```python
from build123d import *

# Parameters (mm, degrees)
SKETCH1_R                = 155.575
SKETCH1_R_2              = 7.9375
BOSS_EXTRUDE1_DEPTH      = 4.7625
FILLET1_R                = 12.7
FILLET4_R                = 2.54
H_0_266_DIAMETER_HOLE1_D = 6.7564


with BuildPart() as part:
    # Sketch1 → Boss-Extrude1 (new body)
    with BuildSketch(Plane.XY):
        Circle(SKETCH1_R)
        with BuildLine():
            ThreePointArc((-125.107792883, -62.16212802), (-120.983748909, 69.85), (-8.719914422, 139.427590858))
            Line((-8.719914422, 139.427590858), (-12.49892387, 7.216257061))
            Line((-12.49892387, 7.216257061), (-125.107792883, -62.16212802))
        make_face(mode=Mode.SUBTRACT)
        with BuildLine():
            ThreePointArc((8.719914422, 139.427590858), (120.983748909, 69.85), (125.107792883, -62.16212802))
            Line((125.107792883, -62.16212802), (12.49892387, 7.216257061))
            Line((12.49892387, 7.216257061), (8.719914422, 139.427590858))
        make_face(mode=Mode.SUBTRACT)
        with BuildLine():
            ThreePointArc((116.38787846, -77.265462838), (0, -139.7), (-116.38787846, -77.265462838))
            Line((-116.38787846, -77.265462838), (0, -14.432514122))
            Line((0, -14.432514122), (116.38787846, -77.265462838))
        make_face(mode=Mode.SUBTRACT)
        with BuildLine():
            Line((-12.585726429, 4.179407795), (-12.694815268, 0.362857143))
            ThreePointArc((-12.694815268, 0.362857143), (-10.998522628, -6.35), (-6.03316413, -11.17546109))
            Line((-6.03316413, -11.17546109), (-2.673389891, -12.98926271))
            Line((-2.673389891, -12.98926271), (-112.467905529, -72.262730545))
            ThreePointArc((-112.467905529, -72.262730545), (-120.983748909, -69.85), (-118.815313164, -61.268698026))
            Line((-118.815313164, -61.268698026), (-12.585726429, 4.179407795))
        make_face(mode=Mode.SUBTRACT)
        with BuildLine():
            ThreePointArc((118.815313164, -61.268698026), (120.983748909, -69.85), (112.467905529, -72.262730545))
            Line((112.467905529, -72.262730545), (2.673389891, -12.98926271))
            Line((2.673389891, -12.98926271), (6.03316413, -11.17546109))
            ThreePointArc((6.03316413, -11.17546109), (10.998522628, -6.35), (12.694815268, 0.362857143))
            Line((12.694815268, 0.362857143), (12.585726429, 4.179407795))
            Line((12.585726429, 4.179407795), (118.815313164, -61.268698026))
        make_face(mode=Mode.SUBTRACT)
        Circle(SKETCH1_R_2, mode=Mode.SUBTRACT)
        with BuildLine():
            ThreePointArc((-6.347407634, 133.531428571), (0, 139.7), (6.347407634, 133.531428571))
            Line((6.347407634, 133.531428571), (9.938137929, 7.907174875))
            ThreePointArc((9.938137929, 7.907174875), (0, 12.7), (-9.938137929, 7.907174875))
            Line((-9.938137929, 7.907174875), (-6.347407634, 133.531428571))
        make_face(mode=Mode.SUBTRACT)
    extrude(amount=-BOSS_EXTRUDE1_DEPTH)

    # Fillet1
    fillet1_edges = [part.edges().sort_by_distance(p)[0] for p in [
        (12.49892387, 7.216257061, -2.38125),
        (0, -14.432514122, -2.38125),
        (-12.49892387, 7.216257061, -2.38125),
    ]]
    fillet(fillet1_edges, radius=FILLET1_R)

    # Fillet4
    fillet4_edges = [part.edges().sort_by_distance(p)[0] for p in [
        (12.585726429, 4.179407795, -2.38125),
        (2.673389891, -12.98926271, -2.38125),
        (-2.673389891, -12.98926271, -2.38125),
        (-12.585726429, 4.179407795, -2.38125),
        (-9.938137929, 7.907174875, -2.38125),
        (9.938137929, 7.907174875, -2.38125),
    ]]
    fillet(fillet4_edges, radius=FILLET4_R)

    # H (0.266) Diameter Hole1 (through all)
    with Locations(Plane.XY):
        with Locations((0, 147.6375), (127.857825551, -73.81875), (-127.857825551, -73.81875)):
            Hole(H_0_266_DIAMETER_HOLE1_D / 2)


solid = part.part
```
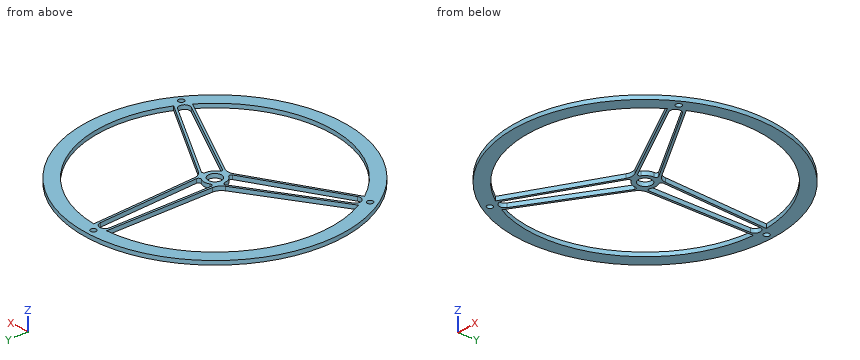
The listing builds one solid part. Answer for the finished solid, in the listing's coordinates (mm). Round coordinates to 2 decimals unless told otherwise and drop trailing zeros. Write each loop counter-clockwise with the first axis right and the second up, starting at its lowest first coordinate (ties: lowest second). Pieces come first, ordered by that corner, then holes. Notation, with made-up numbers: (27, 38) -> (53, 38) arc R20 ccw to (53, 68) -> close; hole circle Ø6 at (84.25, 41.5). An arc over 180 degrees is marked (long way). Answer as a JSON object with one key per item and string values. Group by question number.
Q1. Each of these flat-tipped pins is pushed along its axis until it touches: pin 1 Ø8 at (x, y) = (127.86, -73.82) entering from +Z; pin 2 Ø2 at (x, z) = (34.5, -4) entering from +Y; pin 3 Ø1.5 at (y, z) = (36.5, -1) entering from +X; pin 4 Ø5.5 at (x, y) = (-127.86, -73.82) entering from -Z. Where does it stop, or does it pass through?
Q2. Section D-D (y = 77) is taken. Write down the section's boundary in (x, z), plus the area to 3 significant figures.
Q3. Straight lines are drawn through the part: line 1 along Y through (x, z) = (90.5, -1.6); line 2 along X through (y, z) = (-1, -2.55); line 3 along Y through (x, z) = (-17, -2). For each, find the intervals that lie inside material, in ascending order.
Q4. Section C-C (x = 74.5) is taken. Write down the section's boundary in (y, z).
Q5. Section A-A (x = 135) is taken. Write down the section's boundary in (y, z).
Q6. Section B-B (y = -121.5) is taken. Write down the section's boundary in (x, z), plus the area to 3 significant figures.
Check values:
{
 "1": {"pin 1": "z = 0", "pin 2": "y = 151.93", "pin 3": "x = 151.41", "pin 4": "through"},
 "2": {"outline": "(-135.18, -4.76) -> (-116.56, -4.76) -> (-116.56, 0) -> (-135.18, 0) -> close; (-10.5, -4.76) -> (-7.96, -4.76) -> (-7.96, 0) -> (-10.5, 0) -> close; (7.96, -4.76) -> (10.5, -4.76) -> (10.5, 0) -> (7.96, 0) -> close; (116.56, -4.76) -> (135.18, -4.76) -> (135.18, 0) -> (116.56, 0) -> close", "area": "202 mm^2"},
 "3": {"line 1": "-126.54 to -106.42, -63.29 to -60.4, -43.82 to -40.84, 106.42 to 126.54", "line 2": "-155.57 to -139.7, -25.83 to -20.99, -12.66 to -7.87, 7.87 to 12.66, 20.99 to 25.83, 139.7 to 155.57", "line 3": "-154.64 to -138.66, -23.61 to -20.72, 1.46 to 4.57, 138.66 to 154.64"},
 "4": {"outline": "(-136.58, -4.76) -> (-118.18, -4.76) -> (-118.18, 0) -> (-136.58, 0) -> close; (-54.65, -4.76) -> (-51.77, -4.76) -> (-51.77, 0) -> (-54.65, 0) -> close; (-33.97, -4.76) -> (-30.98, -4.76) -> (-30.98, 0) -> (-33.97, 0) -> close; (118.18, -4.76) -> (136.58, -4.76) -> (136.58, 0) -> (118.18, 0) -> close"},
 "5": {"outline": "(-77.32, -4.76) -> (-35.93, -4.76) -> (-35.93, 0) -> (-77.32, 0) -> close; (35.93, -4.76) -> (77.32, -4.76) -> (77.32, 0) -> (35.93, 0) -> close"},
 "6": {"outline": "(-97.17, -4.76) -> (-68.95, -4.76) -> (-68.95, 0) -> (-97.17, 0) -> close; (68.95, -4.76) -> (97.17, -4.76) -> (97.17, 0) -> (68.95, 0) -> close", "area": "269 mm^2"}
}
